from build123d import *

# Parameters (mm, degrees)
F0_R     = 3.5
F1_DEPTH = 20
F0_W     = 53
F0_H     = 91.5
F0_H_2   = 17
F2_DEPTH = 13


with BuildPart() as f1:
    # F0 (on Front) → F1 (new body)
    with BuildSketch(Plane.XZ):
        with BuildLine():
            Line((-25.671420519, 79.08), (-25.671420519, 157.08))
            Line((-25.671420519, 157.08), (-78.671420519, 157.08))
            Line((-78.671420519, 157.08), (-78.671420519, 104.58))
            ThreePointArc((-78.671420519, 104.58), (-68.671420519, 94.58), (-78.671420519, 84.58))
            Line((-78.671420519, 84.58), (-78.671420519, -4.42))
            Line((-78.671420519, -4.42), (-25.671420519, -4.42))
            Line((-25.671420519, -4.42), (-25.671420519, 59.08))
            Line((-25.671420519, 59.08), (-31.671420519, 59.08))
            ThreePointArc((-31.671420519, 59.08), (-41.671420519, 69.08), (-31.671420519, 79.08))
            Line((-31.671420519, 79.08), (-25.671420519, 79.08))
        make_face()
        with Locations((-47.3698007467, 27.08)):
            Circle(F0_R, mode=Mode.SUBTRACT)
        with Locations((-47.3698007467, 87.08)):
            Circle(F0_R, mode=Mode.SUBTRACT)
        with Locations((-47.3698007467, 147.08)):
            Circle(F0_R, mode=Mode.SUBTRACT)
    extrude(amount=-F1_DEPTH)



with BuildPart() as f1b:
    # F0 (on Front) → F1, piece 2 (new body)
    with BuildSketch(Plane.XZ):
        with BuildLine():
            Line((-25.671420519, -54.42), (-25.671420519, -21.42))
            Line((-25.671420519, -21.42), (-68.7845605524, -21.42))
            ThreePointArc((-68.7845605524, -21.42), (-71.088545075, -29.4392024052), (-78.671420519, -32.92))
            Line((-78.671420519, -32.92), (-78.671420519, -54.42))
            Line((-78.671420519, -54.42), (-25.671420519, -54.42))
        make_face()
        with Locations((-47.171420519, -32.92)):
            Circle(F0_R, mode=Mode.SUBTRACT)
    extrude(amount=-F1_DEPTH)


with BuildPart() as f1c:
    # F0 (on Front) → F1, piece 3 (new body)
    with BuildSketch(Plane.XZ):
        with Locations((-52.171420519, -117.17)):
            Rectangle(F0_W, F0_H)
        with Locations((-47.171420519, -152.92)):
            Circle(F0_R, mode=Mode.SUBTRACT)
        with Locations((-47.171420519, -92.92)):
            Circle(F0_R, mode=Mode.SUBTRACT)
    extrude(amount=-F1_DEPTH)


with BuildPart() as f1_1:
    add(f1.part)

    add(f1b.part)  # F2 merges F1b

    add(f1c.part)  # F2 merges F1c
    # F0 (on Front) → F2 (join)
    with BuildSketch(Plane.XZ):
        with BuildLine():
            Line((-25.671420519, -21.42), (-25.671420519, -4.42))
            Line((-25.671420519, -4.42), (-78.671420519, -4.42))
            Line((-78.671420519, -4.42), (-78.671420519, -12.92))
            ThreePointArc((-78.671420519, -12.92), (-72.1522181138, -15.3371245559), (-68.7845605524, -21.42))
            Line((-68.7845605524, -21.42), (-25.671420519, -21.42))
        make_face()
        with Locations((-56.171420519, -12.92)):
            Circle(F0_R, mode=Mode.SUBTRACT)
        with Locations((-52.171420519, -62.92)):
            Rectangle(F0_W, F0_H_2)
        with Locations((-56.171420519, -62.92)):
            Circle(F0_R, mode=Mode.SUBTRACT)
    extrude(amount=-F2_DEPTH)


solid = f1_1.part
Input: part model. Units: mm. Frame: model coordinates. A direction names the side the tool comes from. Coordinates: 2 decimals unless noted, no trailing zeros. Loops run counter-clockwise (first coordinate to the right, second up) from the corner with the lowest first, then second, coordinate; pieces in that order, holes last. Notation, with made-up numbers: (-36.75, 5.25) - (4.25, 5.25) arc R20 cw to (4.25, 35.25) - close; hole circle Ø5 at (58.5, 78). An arc over 180 degrees is marked (long way). Answer in a Markdown table with one row per item. Add a question column.
Item 1: Section query B-B on y = 5. State how many separate pieces and enclosed holes the cut face has, then the cut area to 3 significant figures.
Item 2: Contact query for a flat-ended pin moving along its axis: P1, Ø6, axis at x = -63.5, z = -18, coming from the +Y side. Output: stop coordinate, or through.
Item 3: Access query for faces 1 (the flat face through (-29, 10, 79.08)), 2 (the cylindrical face through (-44.03, 9.86, 28.13)), 3 (the flat face through (-53, 16, -4.42)). Directions: +Z, -Z, +X, -X, +Y, -Y. A direction counts if a zero-diameter tool reaches every point of the face in a straight line with its end or side. Return the directions, or none.
Item 4: Mould query, pull axis Z, two halves, no side actions, for faces 4 (the flat face through (-53, 10, -162.92)), 5 (the flat face through (-52, 10, 157.08)), 6 (the flat face through (-53, 16, -54.42)), 7 (the flat face through (-25.671, 10, 118)). Classes: released by +Z, released by -Z, zero draft, split by the parting line, or undercut.
Item 5: Line query: line 1 along Z through (x, y) = (-55.5, 8.5) (3 decimals); line 2 along Z through (x, y) = (-31.5, 5); line 3 along Z through (x, y) = (-51, 18.75). Output: solid intervals per line, ascending. Write a range as [from, to].
Item 6: Section query A-A on z = -152.92. Return the cut outline in (x, y).
Item 7: Section query C-C on x = -56.5. Return the cut outline in (y, z).
Item 8: Section query D-D on z = -62.92. Return the cut outline in (x, y), then the cut area to 3 significant figures.
Recorded:
| question | item | result |
|---|---|---|
| 1 | separate pieces | 1 |
| 1 | enclosed holes | 8 |
| 1 | area | 16,100 mm^2 |
| 2 | P1 | y = 13 |
| 3 | face 1 | +X, +Y, -Y |
| 3 | face 2 | +Y, -Y |
| 3 | face 3 | +X, -X, +Y |
| 4 | face 4 | released by -Z |
| 4 | face 5 | released by +Z |
| 4 | face 6 | undercut |
| 4 | face 7 | zero draft |
| 5 | line 1 | [-162.92, -66.355], [-59.485, -16.355], [-9.485, 157.08] |
| 5 | line 2 | [-162.92, 59.08], [79.08, 157.08] |
| 5 | line 3 | [-162.92, -71.42], [-54.42, -21.42], [-4.42, 157.08] |
| 6 | outline | (-78.67, 0) - (-50.67, 0) - (-50.67, 20) - (-78.67, 20) - close; (-43.67, 0) - (-25.67, 0) - (-25.67, 20) - (-43.67, 20) - close |
| 7 | outline | (0, -162.92) - (20, -162.92) - (20, -71.42) - (13, -71.42) - (13, -66.4) - (0, -66.4) - close; (0, -59.44) - (13, -59.44) - (13, -54.42) - (20, -54.42) - (20, -21.42) - (13, -21.42) - (13, -16.4) - (0, -16.4) - close; (0, -9.44) - (13, -9.44) - (13, -4.42) - (20, -4.42) - (20, 157.08) - (0, 157.08) - close |
| 8 | outline | (-78.67, 0) - (-59.67, 0) - (-59.67, 13) - (-78.67, 13) - close; (-52.67, 0) - (-25.67, 0) - (-25.67, 13) - (-52.67, 13) - close |
| 8 | area | 598 mm^2 |
